Here's how the part is built. I have some questions about the finished solid (model axes, mm). A direction names the side the tool comes from. Round coordinates to 2 decimals unless told otherwise and drop trailing zeros. Order: outer loops, then holes, each group sorted by start corner. A loop starts at its lowest first (then second) coordinate and runs counter-clockwise, first axis right, second up. Notation, with made-up numbers: M -6,68.5 L 10,68.5 A17 cw 10,72.5 Z; hole C -14,21 d7. An arc over 180 degrees is marked long. Write item = value, one per line. Start each with the question number.
Item 1: I want a section at C-C, the plane y = 3.75. List the corners of the cut face in (x, z) for me, plus the area to 3 significant figures.
Item 2: Please list where these lines run through material, in increasing order: L1, parallel to Z at x = 0, y = -1.5; L2, parallel to X at y = 0, z = 4; L3, parallel to Y at x = 1, z = 17.
Item 3: I want a section at B-B, the plane x = 0. List the corners of the cut face in (y, z) for me, plus the area to 3 significant figures.
Item 4: We'd pull the mould along Y, two halves only. Please class faces 3 (the face through (0.014, 0.184, -9.545)), 4 (the face through (0, 0, 20)), 5 (the face through (0, 0, 0)), 6 (the face through (0.014, -0.213, -10.045)): pulls with the +Y half, pulls with the -Y half, needs draft (parallel to the pull), parting line crosses it, or undercut.
Item 5: I'm going to push flat-ended pins straight in: P1, Ø6, axis at y = 3, z = -6, coming from the +X side; P2, Ø5, axis at y = 0.5, z = -7.5, coming from the -X side; P3, Ø1.4, axis at x = 1, y = 1, coming from the -Z side. Where does each tip first touch, or does it pass through?
Item 6: I want a section at A-A, the plane y = 0. List the corners of the cut face in (x, z) for me.
Item 7: I want a section at D-D, the plane z = -7. List the corners of the cut face in (x, y) for me.
Item 8: For faces 1 (the face through (1.617, -0.035, 3.33)), 2 (the face through (0.54, 2.44, 10.14)), which set-ups out of +Z, -Z, +X, -X, +Y, -Y let a thin tool reach every point of the face, with its end or its side?
```python
from build123d import *

# Parameters (mm, degrees)
F0_W     = 2.5
F0_H     = 20
F2_R     = 1.75
F3_DEPTH = 2.5
F5_DEPTH = 1


with BuildPart() as f1:
    # F0 (on Front) → F1 (revolve)
    with BuildSketch(Plane.XZ):
        with Locations((-1.25, 10)):
            Rectangle(F0_W, F0_H)
    revolve(axis=Axis((0, 0, 10), (0, 0, 1)))

    # F2 (on Front) → F3 (cut, symmetric)
    with BuildSketch(Plane.XZ):
        with Locations((0, 4)):
            Circle(F2_R)
    extrude(amount=F3_DEPTH, both=True, mode=Mode.SUBTRACT)

    # F4 (on Right) → F5 (join, symmetric)
    with BuildSketch(Plane.YZ):
        with BuildLine():
            ThreePointArc((2.244925, 0), (-0.005075, -9.548809), (-2.255075, 0))
            Line((-2.255075, 0), (-2.478312, 0.447398))
            ThreePointArc((-2.478312, 0.447398), (-0.005075, -10.048809), (2.468162, 0.447398))
            Line((2.468162, 0.447398), (2.244925, 0))
        make_face()
    extrude(amount=F5_DEPTH, both=True)


solid = f1.part
```
Filled in:
q1.outline = M -1,-8.58 L 1,-8.58 L 1,-7.87 L -1,-7.87 Z; M -1,-1.15 L 1,-1.15 L 1,-0.44 L -1,-0.44 Z
q1.area = 2.85 mm^2
q2.L1 = -9.84 to -9.32, 0 to 2.25, 5.75 to 20
q2.L2 = -2.5 to -1.75, 1.75 to 2.5
q2.L3 = -2.29 to 2.29
q3.outline = M -2.5,0.44 A5.54 ccw long 2.5,0.43 L 2.5,2.25 L -2.5,2.25 Z; M -2.5,5.75 L 2.5,5.75 L 2.5,20 L -2.5,20 Z; hole M -2.26,0 A5.04 ccw long 2.24,0 Z
q3.area = 96.5 mm^2
q4.face_3 = undercut
q4.face_4 = needs draft
q4.face_5 = undercut
q4.face_6 = parting line crosses it
q5.P1 = 1
q5.P2 = -1
q5.P3 = -10.04
q6.outline = M -2.5,0 L 2.5,0 L 2.5,20 L -2.5,20 Z; M -1,-10.05 L 1,-10.05 L 1,-9.55 L -1,-9.55 Z; hole C 0,4 d3.5
q7.outline = M -1,-4.95 L 1,-4.95 L 1,-4.39 L -1,-4.39 Z; M -1,4.38 L 1,4.38 L 1,4.94 L -1,4.94 Z
q8.face_1 = +Y, -Y
q8.face_2 = +Z
